Geometry: final body of the model. Coordinates: model frame, mm. Coordinates: 2 decimals unless noted, no trailing zeros. Loops run counter-clockwise (first coordinate to the right, second up) from the corner with the lowest first, then second, coordinate; pieces in that order, holes last. Notation, with made-up numbers: (41.25, 0) - (56.25, 0) arc R23 cw to (56.25, 32) - close; hole circle Ø2 at (86.25, 67.25). An arc over 180 degrees is marked (long way). Answer in a Markdown table with one row per item.
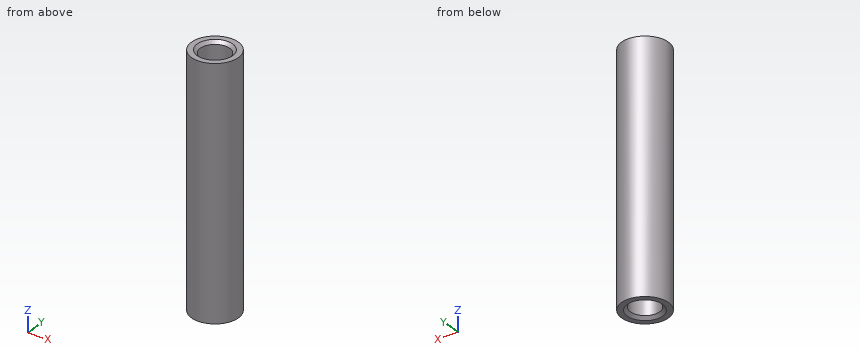
from build123d import *

# Parameters (mm, degrees)
ESBO_O1_R                = 4
RESSALTO_EXTRUS_O1_DEPTH = 21


with BuildPart() as part:
    # Esboço1 → Ressalto-extrusão1 (new, symmetric)
    with BuildSketch(Plane.XY):
        with Locations(Location((0, 0, 0), (0, 0, 180))):
            Circle(ESBO_O1_R)
    extrude(amount=RESSALTO_EXTRUS_O1_DEPTH, both=True)

    # Esboço3 → Furo roscado de M61 (revolve, cut)
    with BuildSketch(Plane(origin=(0, 0, 21), x_dir=(0, -1, 0), z_dir=(1, 0, 0))):
        Polygon((0, 0), (0, 16.502151548), (2.5, 15), (2.5, 0.525), (3.025, 0), align=None)
    furo_roscado_de_m61 = revolve(axis=Axis((0, 0, 27.35), (0, 0, -1)), mode=Mode.SUBTRACT)

    # Espelhar2: Furo roscado de M61 across plane
    add(furo_roscado_de_m61.mirror(Plane.XY), mode=Mode.SUBTRACT)


solid = part.part
(1) Ray query, probe 1 along Y at (x, z) = (0, -10.5); probe 2 along X at (y, z) = (2.25, -17.5); probe 3 along X at (y, z) = (0.5, 8). Return the intervals inside material, ascending.
Verdict:
| item | result |
|---|---|
| probe 1 | y = -4 to -2.5, 2.5 to 4 |
| probe 2 | x = -3.31 to -1.09, 1.09 to 3.31 |
| probe 3 | x = -3.97 to -2.45, 2.45 to 3.97 |
(2) First-contact query: pin 1 Ø3 at (x, z) = (2, 16.5) entering from -Y; pin 2 Ø1.5 at (y, z) = (1, -8.5) entering from +X; pin 3 Ø4.5 at (x, y) = (0, 0) entering from +Z; pin 4 Ø3 at (x, y) = (-2, 1.5) entering from +Z. Flat tips, straight axial feed; report the tip coordinate or a pass-through.
Verdict:
| item | result |
|---|---|
| pin 1 | stops at y = -3.97 |
| pin 2 | stops at x = 3.99 |
| pin 3 | stops at z = 5.85 |
| pin 4 | stops at z = 21 |
(3) Cut plane B-B on z = 0. Output: boundary loops of the cut face in (x, y), then the cut area to 3 significant figures.
Verdict:
| item | result |
|---|---|
| outline | circle Ø8 at (0, 0) |
| area | 50.3 mm² |
(4) Cut plane A-A on z = -11.5. Output: boundary loops of the cut face in (x, y), then the cut area to 3 significant figures.
Verdict:
| item | result |
|---|---|
| outline | circle Ø8 at (0, 0); hole circle Ø5 at (0, 0) |
| area | 30.6 mm² |
(5) Cut plane C-C on y = 3.5. Output: boundary loops of the cut face in (x, z), then the cut area to 3 significant figures.
Verdict:
| item | result |
|---|---|
| outline | (-1.94, -21) - (1.94, -21) - (1.94, 21) - (-1.94, 21) - close |
| area | 163 mm² |
